Build history of the part. All positions in model axes, mm. A direction names the side the tool comes from. Coordinates: 2 decimals unless noted, no trailing zeros. Order: outer loops, then holes, each group sorted by start corner. A loop starts at its lowest first (then second) coordinate and runs counter-clockwise, first axis right, second up. Notation, with made-up numbers: M -39.5,66 L -32.5,66 A26 ccw -32.5,93 Z; hole C -28,50.25 d10. An arc over 180 degrees is marked long. Write item = value, one per line. Start each with the question number.
Q1. Band-saw the part on C-C on x = -88. Write the cut outline in (y, z).
Q2. Drill centre lines: probe 1 along Z at (x, y) = (40, 3.5); probe 2 along X at (y, z) = (8.75, -109.5); probe 3 along Y at (x, z) = (-113.45, 0). Where is each one in solid material? Low to high.
Q3. Band-saw the part on A-A on x = 62. Write the cut outline in (y, z), plus the area to 4 significant figures.
Q4. 3-axis set-ups, long thin cutter, end or side, ignore diameter. For faces 1 (the face through (31.25, 6, 0)), 2 (the face through (-2, 10, -175)), 3 (the face through (114.788, 14.957, -0.651)), 4 (the face through (-114.788, 14.957, -0.651)): which of +Z, -Z, +X, -X, +Y, -Y reach the whole face in a straight line?
Q5. Band-saw the part on B-B on z = 0. Write the cut outline in (x, y), plus the area to 4 significant figures.
Q6. Pin check, flat tips, straight feed: P1, Ø6, axis at y = 10, z = 0, coming from the +X side; P2, Ø8, axis at x = 79, z = -55, coming from the +Y side; P3, Ø3, axis at y = 8, z = -0.5, coming from the -X side. Stop position of each tip, or through.
Q7. Pull direction X, two halves, no side cores. Call faces 5 (the face through (-112, 10, 0)), 6 (the face through (-2, 10, 175)), 7 (the face through (102.5, 6, 2)), 8 (the face through (-1, 17.5, -2)): released by +X, released by -X, zero draft, split by the parting line, or undercut.
Q8. Band-saw the part on D-D on z = -61.5. Write the cut outline in (x, y).
```python
from build123d import *

# Parameters (mm, degrees)
SKETCH1_W                = 235
SKETCH1_H                = 350
SKETCH1_W_2              = 205
SKETCH1_H_2              = 320
BOSS_EXTRUDE1_DEPTH      = 20
BOSS_EXTRUDE2_START      = 15
SKETCH1_2_W              = 205
SKETCH1_2_H              = 320
BOSS_EXTRUDE2_DEPTH      = 2.5
BOSS_EXTRUDE2_DEPTH_BACK = 2.5
SKETCH2_W                = 40
SKETCH2_H                = 50
BOSS_EXTRUDE3_DEPTH      = 12.5
SKETCH3_R                = 5
CUT_EXTRUDE1_DEPTH       = 5.5
CUT_EXTRUDE2_START       = -235
SKETCH3_3_R              = 5
CUT_EXTRUDE2_DEPTH       = 5.5


with BuildPart() as part:
    # Sketch1 → Boss-Extrude1 (new body)
    with BuildSketch(Plane(origin=(0, 0, 0), x_dir=(1, 0, 0), z_dir=(0, 1, 0))):
        Rectangle(SKETCH1_W, SKETCH1_H)
        Rectangle(SKETCH1_W_2, SKETCH1_H_2, mode=Mode.SUBTRACT)
    extrude(amount=BOSS_EXTRUDE1_DEPTH)

    # Sketch1<2> → Boss-Extrude2 (add, two sides)
    with BuildSketch(Plane(origin=(0, 0, 0), x_dir=(1, 0, 0), z_dir=(0, 1, 0)).offset(BOSS_EXTRUDE2_START)) as boss_extrude2_sk:
        Rectangle(SKETCH1_2_W, SKETCH1_2_H)
    extrude(amount=BOSS_EXTRUDE2_DEPTH)
    extrude(boss_extrude2_sk.sketch, amount=-BOSS_EXTRUDE2_DEPTH_BACK)

    # Sketch2 → Boss-Extrude3 (add)
    with BuildSketch(Plane.XZ.offset(-12.5)):
        with Locations((51.25, 0)):
            Rectangle(SKETCH2_W, SKETCH2_H)
    extrude(amount=BOSS_EXTRUDE3_DEPTH)

    # Sketch3 → Cut-Extrude1 (cut)
    with BuildSketch(Plane.ZY.offset(117.5)):
        with Locations((0, 10)):
            Circle(SKETCH3_R)
    extrude(amount=-CUT_EXTRUDE1_DEPTH, mode=Mode.SUBTRACT)

    # Sketch3<3> → Cut-Extrude2 (cut)
    with BuildSketch(Plane.ZY.offset(117.5).offset(CUT_EXTRUDE2_START)):
        with Locations((0, 10)):
            Circle(SKETCH3_3_R)
    extrude(amount=CUT_EXTRUDE2_DEPTH, mode=Mode.SUBTRACT)


solid = part.part
```
Recorded:
q1.outline = M 0,-175 L 20,-175 L 20,-160 L 17.5,-160 L 17.5,160 L 20,160 L 20,175 L 0,175 L 0,160 L 12.5,160 L 12.5,-160 L 0,-160 Z
q2.probe_1 = -175 to -160, -25 to 25, 160 to 175
q2.probe_2 = -117.5 to -102.5, 102.5 to 117.5
q2.probe_3 = 0 to 5, 15 to 20
q3.outline = M 0,-175 L 20,-175 L 20,-160 L 17.5,-160 L 17.5,160 L 20,160 L 20,175 L 0,175 L 0,160 L 12.5,160 L 12.5,25 L 0,25 L 0,-25 L 12.5,-25 L 12.5,-160 L 0,-160 Z
q3.area = 2,825 mm2
q4.face_1 = -Y
q4.face_2 = -Z, +X, -X, +Y, -Y
q4.face_3 = +X
q4.face_4 = -X
q5.outline = M -117.5,0 L -102.5,0 L -102.5,12.5 L 31.25,12.5 L 31.25,0 L 71.25,0 L 71.25,12.5 L 102.5,12.5 L 102.5,0 L 117.5,0 L 117.5,5 L 112,5 L 112,15 L 117.5,15 L 117.5,20 L 102.5,20 L 102.5,17.5 L -102.5,17.5 L -102.5,20 L -117.5,20 L -117.5,15 L -112,15 L -112,5 L -117.5,5 Z
q5.area = 2,015 mm2
q6.P1 = 112
q6.P2 = 17.5
q6.P3 = -112
q7.face_5 = released by -X
q7.face_6 = zero draft
q7.face_7 = undercut
q7.face_8 = undercut
q8.outline = M -117.5,0 L -102.5,0 L -102.5,12.5 L 102.5,12.5 L 102.5,0 L 117.5,0 L 117.5,20 L 102.5,20 L 102.5,17.5 L -102.5,17.5 L -102.5,20 L -117.5,20 Z
